Geometry check sheet. Reference: the model listing, model coordinates, mm. A direction names the side the tool comes from. Round coordinates to 2 decimals unless told otherwise and drop trailing zeros. Loops run counter-clockwise (first coordinate to the right, second up) from the corner with the lowest first, then second, coordinate; pieces in that order, holes last.
```python
from build123d import *

# Parameters (mm, degrees)
BOSS_EXTRUDE1_DEPTH = 1
FILLET1_R           = 0.2
SKETCH2_R           = 2
BOSS_EXTRUDE2_DEPTH = 6.7
CHAMFER1_SIZE       = 0.5
FILLET2_R           = 0.2


with BuildPart() as part:
    # Sketch1 → Boss-Extrude1 (new, symmetric)
    with BuildSketch(Plane(origin=(0, 0, 0), x_dir=(0, 0, -1), z_dir=(1, 0, 0))):
        Polygon((2.5, 1.443375673), (0, 2.886751346), (-2.5, 1.443375673), (-2.5, -1.443375673), (0, -2.886751346), (2.5, -1.443375673), align=None)
    extrude(amount=BOSS_EXTRUDE1_DEPTH, both=True)

    # Fillet1
    fillet1_edges = [part.edges().sort_by_distance(p)[0] for p in [
        (1, 2.165063509, 1.25),
        (1, 0, 2.5),
        (1, -2.165063509, 1.25),
        (1, -2.165063509, -1.25),
        (1, 0, -2.5),
        (-1, -2.165063509, -1.25),
        (-1, -2.165063509, 1.25),
        (-1, 0, 2.5),
        (-1, 2.165063509, 1.25),
        (-1, 2.165063509, -1.25),
        (-1, 0, -2.5),
        (1, 2.165063509, -1.25),
    ]]
    fillet(fillet1_edges, radius=FILLET1_R)

    # Sketch2 → Boss-Extrude2 (add)
    with BuildSketch(Plane.ZY.offset(1)):
        with Locations(Location((0, 0, 0), (0, 0, 180))):
            Circle(SKETCH2_R)
    extrude(amount=BOSS_EXTRUDE2_DEPTH)

    # Chamfer1
    chamfer1_edges = [part.edges().sort_by_distance(p)[0] for p in [
        (-7.7, 0, 2),
    ]]
    chamfer(chamfer1_edges, length=CHAMFER1_SIZE)

    # Fillet2
    fillet2_edges = [part.edges().sort_by_distance(p)[0] for p in [
        (-1, 0, 2),
    ]]
    fillet(fillet2_edges, radius=FILLET2_R)


solid = part.part
```
1) Access from +Z, -Z, +X, -X, +Y, -Y to the whole of each face (thin tool, end or side, straight path). Record for faces 1 (the face through (0.011, -2.155, 1.267)), 2 (the face through (-4, 2, 0)).
Report:
face 1: +Z, +X, -X, -Y
face 2: -X
2) Sectioned sample at A-A, the plane x = -0.25. Record the cut outline in (y, z), then the cut area to 3 significant figures.
Report:
outline: (-2.89, 0) - (-1.44, -2.5) - (1.44, -2.5) - (2.89, 0) - (1.44, 2.5) - (-1.44, 2.5) - close
area: 21.7 mm2
3) Sectioned sample at B-B, the plane y = 0. Record the cut outline in (x, z).
Report:
outline: (-7.7, -1.5) - (-7.2, -2) - (-1.2, -2) arc R0.2 cw to (-1, -2.2) - (-1, -2.3) arc R0.2 ccw to (-0.8, -2.5) - (0.8, -2.5) arc R0.2 ccw to (1, -2.3) - (1, 2.3) arc R0.2 ccw to (0.8, 2.5) - (-0.8, 2.5) arc R0.2 ccw to (-1, 2.3) - (-1, 2.2) arc R0.2 cw to (-1.2, 2) - (-7.2, 2) - (-7.7, 1.5) - close
4) Sectioned sample at C-C, the plane x = -2.5. Record the cut outline in (y, z), then the cut area to 3 significant figures.
Report:
outline: circle Ø4 at (0, 0)
area: 12.6 mm2
5) Gauge pin test, flat ends, axial feed: pin 1 (3 mm diameter, centred on x = -5, y = 1.5, fed in from +Z); pin 2 (1.5 mm diameter, centred on x = -2.5, z = -1, fed in from -Y); pin 3 (1 mm diameter, centred on x = -0.5, z = -1, fed in from +Y). Record the tip position at first contact, or that the pin passes through.
Report:
pin 1: stops at z = 2
pin 2: stops at y = -1.98
pin 3: stops at y = 2.6
6) Scan lines: line 1 along X through (y, z) = (2.35, -0.3); line 2 along Y through (x, z) = (-1.5, 1.15); line 3 along Z through (x, y) = (0, -2.25). Record each from-to range of solid material in increasing order.
Report:
line 1: x = -1 to 1
line 2: y = -1.64 to 1.64
line 3: z = -1.1 to 1.1
